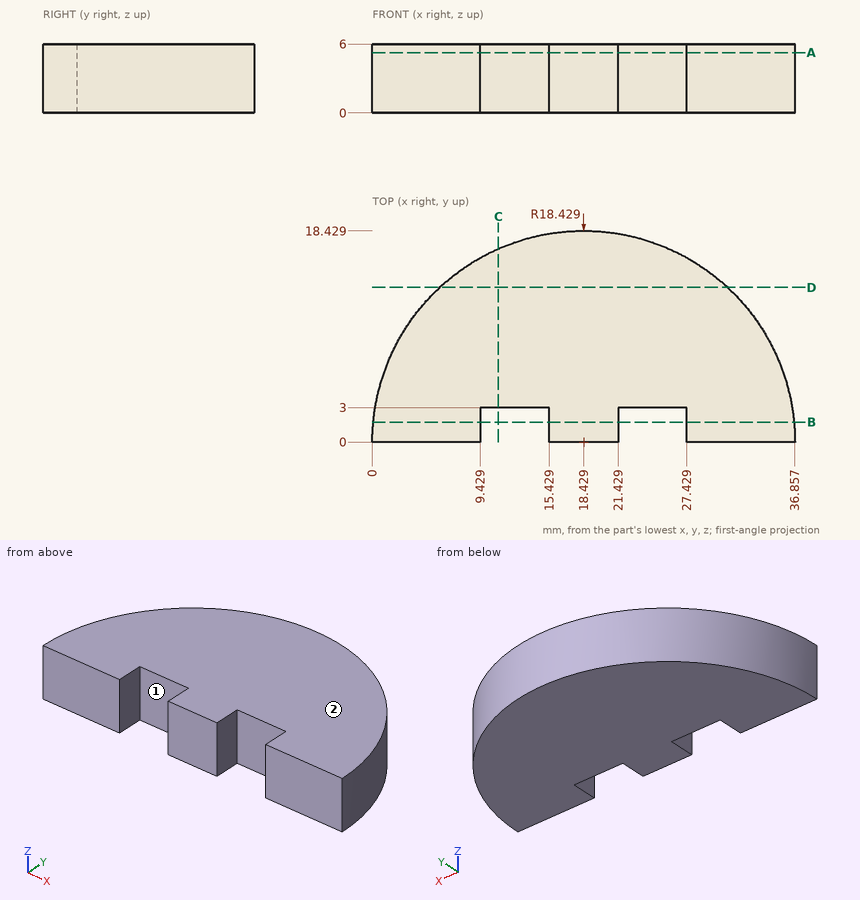
The drawing under review shows one solid part. Ordinate dimensions are in mm from its lowest x, y, z. A direction names the side the tool comes from. Coordinates: 2 decimals unless noted, no trailing zeros. Loops run counter-clockwise (first coordinate to the right, second up) from the corner with the lowest first, then second, coordinate; pieces in that order, holes last. Notation, with made-up numbers: (-22.5, -31) - (20.5, -31) arc R33 ccw to (20.5, 7) - close; hole circle Ø1 at (19, 3). An arc over 180 degrees is marked (long way). Return JSON: item names as keys, results as strings.
Item 1: Take a section at A-A (z = 5.25). Give the boundary of the cut face in (x, y).
Determined:
{"outline": "(0, 0) - (9.43, 0) - (9.43, 3) - (15.43, 3) - (15.43, 0) - (21.43, 0) - (21.43, 3) - (27.43, 3) - (27.43, 0) - (36.86, 0) arc R18.43 ccw to start"}
Item 2: Take a section at C-C (x = 11). Give the boundary of the cut face in (y, z) (1 decimal), then the cut area to 3 significant figures.
Determined:
{"outline": "(3, 0) - (16.9, 0) - (16.9, 6) - (3, 6) - close", "area": "83.2 mm2"}
Item 3: Take a section at D-D (y = 13.5). Give the boundary of the cut face in (x, z) (1 decimal).
Determined:
{"outline": "(5.9, 0) - (31, 0) - (31, 6) - (5.9, 6) - close"}
Item 4: For the marked faces 1 and 2, list the 3-axis set-ups (+Z, -Z, +X, -X, +Y, -Y) from which the entire face can be reached by the end or side of a thin tool; tool diameter is ignored.
Determined:
{"face 1": "+Z, -Z, -Y", "face 2": "+Z, +X, -X, +Y, -Y"}
Item 5: For line 1 (X direction, y = 2.25, z = 5.4); line 2 (X direction, y = 1, z = 5.5); line 3 (Y direction, x = 4, z = 1) (1 decimal), list the stretches that pass through material, from the lowest coordinate up.
Determined:
{"line 1": "x = 0.14 to 9.43, 15.43 to 21.43, 27.43 to 36.72", "line 2": "x = 0.03 to 9.43, 15.43 to 21.43, 27.43 to 36.83", "line 3": "y = 0 to 11.5"}
Item 6: Insertion check: pin 1 (1.5 mm diameter, centred on y = 2, z = 3.5, fed in from +X) (1 decimal); pin 2 (2.5 mm diameter, centred on y = 1.5, z = 2.5, fed in from -X); pin 3 (2 mm diameter, centred on x = 21.5, z = 3.5, fed in from +Y). Each pin has a flat end and moves straight along its axis. Give the tip position at first contact, or say it passes through.
Determined:
{"pin 1": "stops at x = 36.8", "pin 2": "stops at x = 0", "pin 3": "stops at y = 18.31"}
Item 7: Take a section at B-B (y = 1.75). Give the boundary of the cut face in (x, z).
Determined:
{"outline": "(0.08, 0) - (9.43, 0) - (9.43, 6) - (0.08, 6) - close; (15.43, 0) - (21.43, 0) - (21.43, 6) - (15.43, 6) - close; (27.43, 0) - (36.77, 0) - (36.77, 6) - (27.43, 6) - close"}
